Part model, mm, in its own coordinate system. A direction names the side the tool comes from. Give positions to 0.01 mm unless a question says otherwise; leave off trailing zeros. Order: outer loops, then holes, each group sorted by start corner. A loop starts at its lowest first (then second) coordinate and runs counter-clockwise, first axis right, second up. Notation, with made-up numbers: (43, 35) -> (91, 35) arc R22 ccw to (91, 48) -> close; hole circle Ø10 at (40.5, 42). An arc over 180 degrees is marked (long way). Write item = value, one per line. Start each with the question number.
(1) Saw through at C-C, the plane z = 556.5. List the corners of the cut face in (x, y).
(2) Flat gauge pins, fed straight in: pin 1 (12 mm diameter, centred on y = 67.5, z = 269, fed in from -X); pin 2 (3 mm diameter, centred on x = 240.5, y = 45, fed in from -Z); pin 3 (11 mm diameter, centred on y = 14, z = 410, fed in from +X); pin 4 (4 mm diameter, centred on x = 232, z = 303.5, fed in from +Y). Where does each tip first touch, or does it go through?
(3) Saw through at B-B, the plane x = 306. List the corners of the cut face in (y, z), then the cut area to 3 significant figures.
(4) Saw through at D-D, the plane y = 22. List the corners of the cut face in (x, z).
(5) Two-plate mould, pull along Z, no slides. Class faces 1 (the flat face through (345.5, 45.26, 560.7)), 2 (the flat face through (123, 43, 610)), 3 (the cylindrical face through (-14.08, 23.4, 309.44)), 4 (the flat face through (129, 43, 0)): pulls with the +Z half, pulls with the -Z half, needs draft (parallel to the pull), parting line crosses it, or undercut.
(6) Probe line 1 along Z through (x, y) = (262.5, 75); line 2 along Y through (x, z) = (131, 49); line 3 along Y through (x, z) = (34.5, 318). List the from-to ranges inside material, lowest first. Write a range as from..to.
(7) Which spindle directions (+Z, -Z, +X, -X, +Y, -Y) get a long thin tool onto all of the face, cutting with end or side? Do faces 5 (the cylindrical face through (128.952, 87.355, 560.7)), 6 (the cylindrical face through (-73.6, 34.99, 549.59)), 7 (the flat face through (123, 66, 510)), 8 (the flat face through (342.175, 15, 301)), 9 (the flat face through (171, -2.611, 301)). Say none if no direction does.
from build123d import *

# Parameters (mm, degrees)
BOSS_EXTRUDE1_DEPTH = 610
CUT_EXTRUDE1_DEPTH  = 610
CUT_EXTRUDE2_DEPTH  = 703.283548499
BOSS_EXTRUDE2_DEPTH = 100
BOSS_EXTRUDE3_START = -100
BOSS_EXTRUDE3_DEPTH = 100
CUT_REVOLVE3_ANGLE  = 106


with BuildPart() as part:
    # Sketch1 → Boss-Extrude1 (new body)
    with BuildSketch(Plane.XY):
        Polygon((-89.824548177, 33.388821274), (-89.824548177, -2.611178726), (342.175451823, -2.611178726), (342.175451823, 33.388821274), (342.175451823, 63.388821274), (-89.824548177, 63.388821274), align=None)
    extrude(amount=BOSS_EXTRUDE1_DEPTH)

    # Sketch2 → Cut-Extrude1 (cut)
    with BuildSketch(Plane(origin=(0, 63.388821274, 0), x_dir=(1, 0, 0), z_dir=(0, 1, 0))):
        with BuildLine():
            Line((-89.824548177, 0), (-89.824548177, -610))
            ThreePointArc((-89.824548177, -610), (-14.065137005, -305), (-89.824548177, 0))
        make_face()
    extrude(amount=-CUT_EXTRUDE1_DEPTH, mode=Mode.SUBTRACT)

    # Sketch3 → Cut-Extrude2 (cut, through all)
    with BuildSketch(Plane.XY.offset(610)):
        with BuildLine():
            Line((-89.824548177, 30.388821274), (-89.824548177, 63.388821274))
            Line((-89.824548177, 63.388821274), (342.175451823, 63.388821274))
            Line((342.175451823, 63.388821274), (342.175451823, 33.388821274))
            ThreePointArc((342.175451823, 33.388821274), (125.963985264, 62.340005792), (-89.824548177, 30.388821274))
        make_face()
    extrude(amount=-CUT_EXTRUDE2_DEPTH, mode=Mode.SUBTRACT)

    # Sketch4 → Boss-Extrude2 (add)
    with BuildSketch(Plane.XY.offset(610)):
        with BuildLine():
            Line((-96.902742964, 54.365876109), (-89.824548177, 30.388821274))
            ThreePointArc((-89.824548177, 30.388821274), (125.963985264, 62.340005792), (342.175451823, 33.388821274))
            Line((342.175451823, 33.388821274), (348.919965355, 57.461867139))
            ThreePointArc((348.919965355, 57.461867139), (125.790378339, 87.339402998), (-96.902742964, 54.365876109))
        make_face()
    extrude(amount=-BOSS_EXTRUDE2_DEPTH)

    # Sketch5 → Boss-Extrude3 (add)
    with BuildSketch(Plane(origin=(0, 0, 0), x_dir=(-1, 0, 0), z_dir=(0, 0, -1)).offset(BOSS_EXTRUDE3_START)):
        with BuildLine():
            Line((-348.919965355, 57.461867139), (-342.175451823, 33.388821274))
            ThreePointArc((-342.175451823, 33.388821274), (-125.963985264, 62.340005792), (89.824548177, 30.388821274))
            Line((89.824548177, 30.388821274), (96.902742964, 54.365876109))
            ThreePointArc((96.902742964, 54.365876109), (-125.790378339, 87.339402998), (-348.919965355, 57.461867139))
        make_face()
    extrude(amount=BOSS_EXTRUDE3_DEPTH)

    # Sketch6 → Cut-Revolve3 (revolve, cut)
    with BuildSketch(Plane(origin=(-74.37222514, -21.955202584, 0), x_dir=(0, 0, 1), z_dir=(-0.9590821933998281, -0.2831277914712271, 0))):
        with BuildLine():
            Line((100, 79.577203308), (510, 79.577203308))
            ThreePointArc((510, 79.577203308), (305, 294.560025587), (100, 79.577203308))
        make_face()
    revolve(axis=Axis((-96.902742964, 54.365876109, 100), (0, 0, -1)), revolution_arc=CUT_REVOLVE3_ANGLE, mode=Mode.SUBTRACT)


solid = part.part
Results list:
q1.outline = (-96.9, 54.37) -> (-89.82, 30.39) arc R781.32 cw to (-64.54, 37.39) -> (-64.54, -2.61) -> (342.18, -2.61) -> (342.18, 33.39) -> (348.92, 57.46) arc R806.32 ccw to start
q2.pin_1 = 114.24
q2.pin_2 = 0
q2.pin_3 = 342.18
q2.pin_4 = 56.11
q3.outline = (-2.61, 0) -> (68.23, 0) -> (68.23, 100) -> (42.6, 100) -> (42.6, 510) -> (68.23, 510) -> (68.23, 610) -> (-2.61, 610) -> close
q3.area = 32,700 mm^2
q4.outline = (-89.82, 0) -> (342.18, 0) -> (342.18, 610) -> (-89.82, 610) arc R651.83 cw to start
q5.face_1 = needs draft
q5.face_2 = pulls with the +Z half
q5.face_3 = undercut
q5.face_4 = pulls with the -Z half
q6.line_1 = 0..100, 510..610
q6.line_2 = -2.61..87.36
q6.line_3 = -2.61..55.39
q7.face_5 = +Z, -Z, +Y
q7.face_6 = -Y
q7.face_7 = +Y
q7.face_8 = +Z, -Z, +X, -Y
q7.face_9 = +Z, -Z, +X, -X, -Y
